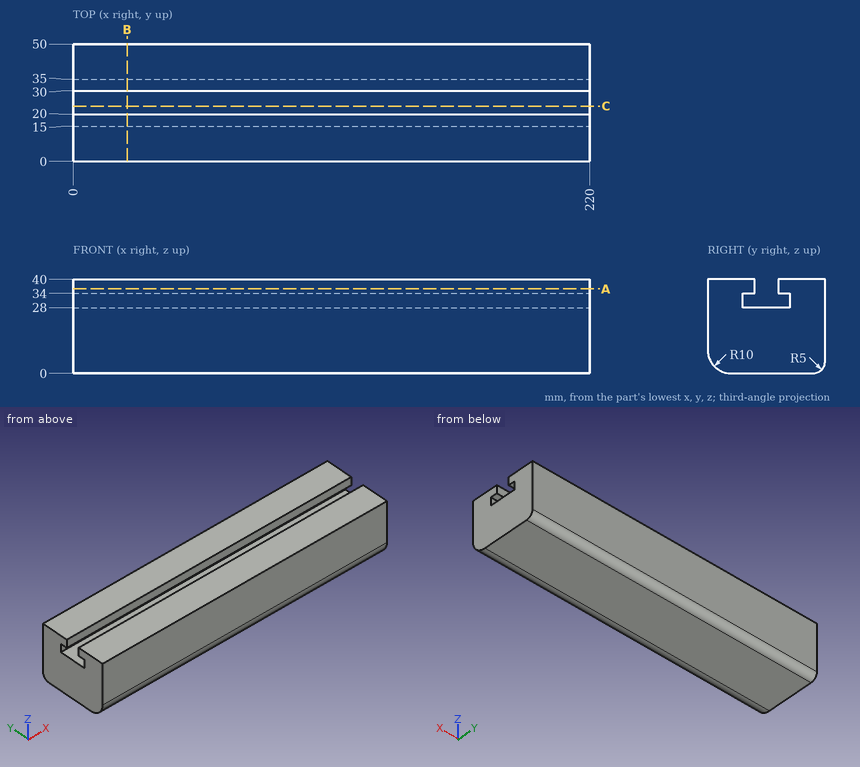
Source: three-view drawing plus pictorial views. Frame: mm from the lowest corner of the part. Round coordinates to 2 decimals unless told otherwise and drop trailing zeros. Write each loop counter-clockwise with the first axis right and the second up, starting at its lowest first coordinate (ties: lowest second). Pieces come first, ordered by that corner, then holes. Notation, with made-up numbers: M 56,-27.5 L 62,-27.5 A21 ccw 62,-12.5 Z; hole C 42,-30.75 d2. An arc over 180 degrees is marked long. Write item = value, one per line.
Item 1: Material intervals for line 1 along Z through (x, y) = (201, 17.5); line 2 along Y through (x, z) = (124.5, 37); line 3 along Y through (x, z) = (123.5, 32.5), sorted ascending. Write a range as [from, to].
Findings:
line_1 = [0, 28], [34, 40]
line_2 = [0, 20], [30, 50]
line_3 = [0, 15], [35, 50]
Item 2: Section query B-B on x = 23. Return loops of the section in (y, z).
Findings:
outline = M 0,10 A10 ccw 10,0 L 45,0 A5 ccw 50,5 L 50,40 L 30,40 L 30,34 L 35,34 L 35,28 L 15,28 L 15,34 L 20,34 L 20,40 L 0,40 Z
Item 3: Section query C-C on y = 23.5. Return loops of the section in (x, z), then the cut area to 3 significant figures.
Findings:
outline = M 0,0 L 220,0 L 220,28 L 0,28 Z
area = 6,160 mm^2
Item 4: Pin query (flat end, axial travel): P1, Ø3, axis at y = 28, z = 5.5, coming from the -X side. Return the tip coordinate at first contact, or that it passes through.
Findings:
P1 = 0
Item 5: Section query A-A on z = 36. Return loops of the section in (x, y), then the cut area to 3 significant figures.
Findings:
outline = M 0,0 L 220,0 L 220,20 L 0,20 Z; M 0,30 L 220,30 L 220,50 L 0,50 Z
area = 8,800 mm^2
